```python
from build123d import *

# Parameters (mm, degrees)
BOSS_EXTRUDE1_DEPTH = 4
SKETCH2_R           = 10
BOSS_EXTRUDE2_DEPTH = 4
SKETCH6_R           = 6
BOSS_EXTRUDE3_DEPTH = 4
SKETCH9_W           = 12
SKETCH9_H           = 12
BOSS_EXTRUDE4_DEPTH = 4


with BuildPart() as part:
    # Sketch1 → Boss-Extrude1 (new body)
    with BuildSketch(Plane.XY):
        Polygon((0, -10), (10, -10), (26, 0), (40, 0), (50, 10), (40, 15), (10, 15), (0, 5), align=None)
    extrude(amount=BOSS_EXTRUDE1_DEPTH)

    # Sketch2 → Boss-Extrude2 (add)
    with BuildSketch(Plane.XY):
        with Locations((50, 10)):
            Circle(SKETCH2_R)
    extrude(amount=BOSS_EXTRUDE2_DEPTH)

    # Sketch6 → Boss-Extrude3 (add)
    with BuildSketch(Plane.XY):
        with Locations((32, 5)):
            Circle(SKETCH6_R)
    extrude(amount=BOSS_EXTRUDE3_DEPTH)

    # Sketch9 → Boss-Extrude4 (add)
    with BuildSketch(Plane.XY):
        with Locations((36, 5)):
            Rectangle(SKETCH9_W, SKETCH9_H)
    extrude(amount=BOSS_EXTRUDE4_DEPTH)


solid = part.part
```
Model file for the job. Use its own axes, mm. A direction names the side the tool comes from. Coordinates: 2 decimals unless noted, no trailing zeros. Loops run counter-clockwise (first coordinate to the right, second up) from the corner with the lowest first, then second, coordinate; pieces in that order, holes last. Notation, with made-up numbers: M -29.75,-31.5 L 24.25,-31.5 A19 ccw 24.25,-17.5 Z; hole C 82.5,75 d7. An arc over 180 degrees is marked long. Use CSV: the item, a comma, the result in double quotes. Start each with the question number.
1. Tool access for faces 1 (the flat face through (25, 15, 2)), 2 (the flat face through (40.54, 14.73, 1.97)), 3 (the cylindrical face through (29.312, -0.364, 1.972)): list every direction of +Z, -Z, +X, -X, +Y, -Y with a clear straight run to the whole face (end or side of a thin tool).
2. Flat gauge pins, fed straight in: pin 1 (0.9 mm diameter, centred on y = 1, z = 2, fed in from +X); pin 2 (2 mm diameter, centred on x = 36.5, z = 2, fed in from -Y). Where does each tip first touch, or does it go through?
3. Band-saw the part on B-B, the plane y = 10. List the corners of the cut face in (x, z), then the cut area to 3 significant figures.
4. Probe probe 1 along Y at (x, z) = (37, 1.6); probe 2 along X at (y, z) = (-3.75, 3.05); probe 3 along X at (y, z) = (1, 2). List the from-to ranges inside material, lowest first. Write a range as [from, to].
5. Band-saw the part on A-A, the plane x = 28. List the corners of the cut face in (y, z), then the cut area to 3 significant figures.
Entries:
1,face 1,"+Z, -Z, -X, +Y"
1,face 2,"+Z, -Z, +Y"
1,face 3,"+Z, -Z, -Y"
2,pin 1,"stops at x = 55.19"
2,pin 2,"stops at y = -1"
3,outline,"M 5,0 L 60,0 L 60,4 L 5,4 Z"
3,area,"220 mm2"
4,probe 1,"y = [-1, 15]"
4,probe 2,"x = [0, 20]"
4,probe 3,"x = [0, 42], [45.64, 54.36]"
5,outline,"M 0,0 L 15,0 L 15,4 L 0,4 Z"
5,area,"60.0 mm2"
